Autodesk Inventor part; units mm, degrees
ref_plane "YZ Plane" through (0, 0, 0) normal (1, 0, 0) x (0, 1, 0)
ref_plane "XZ Plane" through (0, 0, 0) normal (0, 1, 0) x (-1, 0, 0)
ref_plane "XY Plane" through (0, 0, 0) normal (0, 0, 1) x (1, 0, 0)
sketch "Sketch1" plane through (0, 0, 0) normal (0, 0, 1) x (1, 0, 0)
  line L0 (0, 0) -> (203.2, 0)
  line L1 (203.2, 0) -> (203.2, -584.2)
  line L2 (203.2, -584.2) -> (0, -584.2)
  line L3 (0, -584.2) -> (0, 0)
  dimension "d0" = 203.2
  dimension "d1" = 584.2
extrude "Extrusion1" add sketch "Sketch1" along normal blind 25.4
sketch "Sketch2" plane through (0, 0, 25.4) normal (0, 0, 1) x (1, 0, 0)
  line L0 (0, -584.2) -> (203.2, -584.2)
  line L1 (0, 0) -> (25.4, 0)
  line L2 (25.4, 0) -> (25.4, -584.2)
  line L3 (25.4, -584.2) -> (0, -584.2)
  line L4 (0, -584.2) -> (0, 0)
  line L5 (203.2, 0) -> (0, 0)
  line L6 (203.2, 0) -> (177.8, 0)
  line L7 (177.8, 0) -> (177.8, -584.2)
  line L8 (177.8, -584.2) -> (203.2, -584.2)
  line L9 (203.2, -584.2) -> (203.2, 0)
  dimension "d4" = 25.4
  dimension "d5" = 25.4
  dimension "d6" = 584.2
extrude "Extrusion2" add sketch "Sketch2" along normal blind 25.4 contours L4 L1 L2 L0 | L7 L5 L9 L0
properties part number "rev1 tube"
Here's how the part is built. I have some questions about the finished solid (model axes, mm). A direction names the side the tool comes from. Coordinates: 2 decimals unless noted, no trailing zeros. Order: outer loops, then holes, each group sorted by start corner. A loop starts at its lowest first (then second) coordinate and runs counter-clockwise, first axis right, second up.
Item 1: I'm going to push a flat-ended pin straight in: pin 1 Ø12.5 at (y, z) = (-420, 44.5) entering from -X. Where does the tip first touch, or does it pass through?
Response values:
pin 1: stops at x = 0
Item 2: Which directions (+Z, -Z, +X, -X, +Y, -Y) give clear straight access to the entire face, cutting with the end or side of a thin tool? Please do faces 1 (the face through (25.4, -288, 38)), 2 (the face through (190, -288, 50.8)).
Response values:
face 1: +Z, +Y, -Y
face 2: +Z, +X, -X, +Y, -Y
Item 3: Thinking about a two-plate mould opening in X: for faces 3 (the face through (177.8, -288, 38)), 4 (the face through (13, -288, 50.8)), 5 (the face through (203.2, -288, 25)), 6 (the face through (0, -296, 25)), which applies, pulls with the +X half, pulls with the -X half, needs draft (parallel to the pull), parting line crosses it, or undercut?
Response values:
face 3: undercut
face 4: needs draft
face 5: pulls with the +X half
face 6: pulls with the -X half
Item 4: If we section it at C-C, the plane x = 77.5: List the corners of the cut face in (y, z) for me, then the cut area to 3 significant figures.
Response values:
outline: (-584.2, 0) - (0, 0) - (0, 25.4) - (-584.2, 25.4) - close
area: 14,800 mm2
Item 5: I need wall thicknesses on probe 1 along X at (y, z) = (-296, 31); probe 2 along Z at (x, y) = (39, -109.5). Which ranges of each line are inside material? Lowest first, please.
Response values:
probe 1: x = 0 to 25.4, 177.8 to 203.2
probe 2: z = 0 to 25.4
Item 6: If we section it at A-A, the plane z = 31.5: List the corners of the cut face in (x, y) for me, then the cut area to 3 significant figures.
Response values:
outline: (0, -584.2) - (25.4, -584.2) - (25.4, 0) - (0, 0) - close; (177.8, -584.2) - (203.2, -584.2) - (203.2, 0) - (177.8, 0) - close
area: 29,700 mm2
Item 7: If we section it at B-B, the plane y = -209: List the corners of the cut face in (x, z) for me, then the cut area to 3 significant figures.
Response values:
outline: (0, 0) - (203.2, 0) - (203.2, 50.8) - (177.8, 50.8) - (177.8, 25.4) - (25.4, 25.4) - (25.4, 50.8) - (0, 50.8) - close
area: 6,450 mm2
